from build123d import *

# Parameters (mm, degrees)
ESQUISSE2_R             = 5
BOSS_EXTRU_2_DEPTH      = 8
ESQUISSE3_W             = 10
ESQUISSE3_H             = 34.323
BOSS_EXTRU_3_DEPTH      = 6
ENL_V_MAT_EXTRU_1_REACH = 139.007
ESQUISSE4_R             = 4


with BuildPart() as part:
    # Esquisse2 → Boss.-Extru.2 (new body)
    with BuildSketch(Plane(origin=(0, 0, 0), x_dir=(-1, 0, 0), z_dir=(0, 0, 1))):
        Polygon((-45, 128.646), (-45, 0), (-5, 0), (0, 0), (0, 64.323), (0, 128.646), (-5.55, 128.646), align=None)
        with Locations(Location((-22.5, 10, 0), (0, 0, 180))):
            Circle(ESQUISSE2_R, mode=Mode.SUBTRACT)
        with Locations((-22.5, 118.646)):
            Circle(ESQUISSE2_R, mode=Mode.SUBTRACT)
    extrude(amount=BOSS_EXTRU_2_DEPTH)

    # Esquisse3 → Boss.-Extru.3 (add)
    with BuildSketch(Plane(origin=(0, 0, 0), x_dir=(-1, 0, 0), z_dir=(0, 0, -1))):
        with Locations((-22.5, -91.4845)):
            Rectangle(ESQUISSE3_W, ESQUISSE3_H)
        with Locations((-22.5, -37.1615)):
            Rectangle(ESQUISSE3_W, ESQUISSE3_H)
    extrude(amount=BOSS_EXTRU_3_DEPTH)

    # Esquisse4 → Enlèv. mat.-Extru.1 (cut, up to next)
    with BuildSketch(Plane.XY.offset(8), mode=Mode.PRIVATE) as enl_v_mat_extru_1_sk1:
        with Locations((10.1018, -28.6106)):
            Circle(ESQUISSE4_R)
    enl_v_mat_extru_1_tool1 = extrude(enl_v_mat_extru_1_sk1.sketch, amount=-ENL_V_MAT_EXTRU_1_REACH, mode=Mode.PRIVATE) & part.part
    # Esquisse4 → Enlèv. mat.-Extru.1 (cut, up to next)
    with BuildSketch(Plane.XY.offset(8), mode=Mode.PRIVATE) as enl_v_mat_extru_1_sk2:
        with Locations((10.1018, -100.0354)):
            Circle(ESQUISSE4_R)
    enl_v_mat_extru_1_tool2 = extrude(enl_v_mat_extru_1_sk2.sketch, amount=-ENL_V_MAT_EXTRU_1_REACH, mode=Mode.PRIVATE) & part.part
    # Esquisse4 → Enlèv. mat.-Extru.1 (cut, up to next)
    with BuildSketch(Plane.XY.offset(8), mode=Mode.PRIVATE) as enl_v_mat_extru_1_sk3:
        with Locations((18.84, -64.323)):
            Circle(ESQUISSE4_R)
    enl_v_mat_extru_1_tool3 = extrude(enl_v_mat_extru_1_sk3.sketch, amount=-ENL_V_MAT_EXTRU_1_REACH, mode=Mode.PRIVATE) & part.part
    add(enl_v_mat_extru_1_tool1.solids().sort_by_distance((10.1018, -28.6106, 8))[0], mode=Mode.SUBTRACT)
    add(enl_v_mat_extru_1_tool2.solids().sort_by_distance((10.1018, -100.0354, 8))[0], mode=Mode.SUBTRACT)
    add(enl_v_mat_extru_1_tool3.solids().sort_by_distance((18.84, -64.323, 8))[0], mode=Mode.SUBTRACT)


solid = part.part
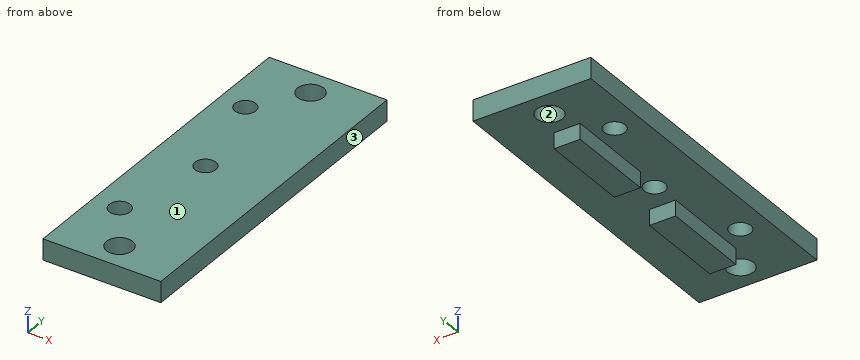
Work out the finished part from the listing and answer in its coordinate system (mm). Face numbers are marked on the shaded views. Round coordinates to 2 decimals unless told otherwise and drop trailing zeros. Order: outer loops, then holes, each group sorted by start corner. A loop starts at its lowest first (then second) coordinate and runs counter-clockwise, first axis right, second up. Notation, with made-up numbers: M 13,-16 L 52,-16 A27 ccw 52,9 Z; hole C 61,56.5 d5. An arc over 180 degrees is marked long. Put each result on its own line as item: value. Start each with the question number.
Q1. Section C-C, the plane y = -35 is taken. Write down the section's boundary in (x, z), and give its area (3 significant figures).
Q2. For a pull along X with two mould halves and no side action, classify the marked faces 1, 2 and 3 as pulls with the +X half, pulls with the -X half, needs draft (parallel to the pull), parting line crosses it, or undercut.
Q3. Section B-B, the plane x = 9 is taken. Write down the section's boundary in (y, z), and give its area (3 significant figures).
Q4. Section A-A, the plane y = -10 is taken. Write down the section's boundary in (x, z), and give its area (3 significant figures).
Q5. Flat-ended cylindrical pins translate along their axes: pin 1 (6.5 mm diameter, centred on y = -44, z = -4, fed in from +X); pin 2 (3 mm diameter, centred on y = -35.5, z = -2.5, fed in from -X); pin 3 (2 mm diameter, centred on x = 8, y = -47, fed in from -Z); pin 4 (10.5 mm diameter, centred on x = 10.1, y = -100.04, fed in from +Z). Find the tip coordinate at first contact, or state that the pin passes through.
Q6. Straight lines are drawn through the part: L1, parallel to Y at x = 18.84, z = 2.75; L2, parallel to Y at x = 13.5, z = 5; L3, parallel to Y at x = 22, z = 1.75. For each, find the intervals that lie inside material, in ascending order. Write a range as [from, to].
Q7. Section D-D, the plane x = 21.5 is taken. Write down the section's boundary in (y, z), and give its area (3 significant figures).
Findings below:
1. outline: M 0,0 L 17.5,0 L 17.5,-6 L 27.5,-6 L 27.5,0 L 45,0 L 45,8 L 0,8 Z
1. area: 420 mm^2
2. face 1: needs draft
2. face 2: undercut
2. face 3: pulls with the +X half
3. outline: M -128.65,0 L -103.88,0 L -103.88,8 L -128.65,8 Z; M -96.19,0 L -32.46,0 L -32.46,8 L -96.19,8 Z; M -24.77,0 L 0,0 L 0,8 L -24.77,8 Z
3. area: 906 mm^2
4. outline: M 0,0 L 17.5,0 L 17.5,8 L 0,8 Z; M 27.5,0 L 45,0 L 45,8 L 27.5,8 Z
4. area: 280 mm^2
5. pin 1: stops at x = 27.5
5. pin 2: stops at x = 17.5
5. pin 3: stops at z = 0
5. pin 4: stops at z = 8
6. L1: y = [-128.65, -122.05], [-115.24, -68.32], [-60.32, -13.41], [-6.59, 0]
6. L2: y = [-128.65, -102.15], [-97.93, -30.72], [-26.5, 0]
6. L3: y = [-128.65, -123.62], [-113.67, -66.78], [-61.87, -14.97], [-5.03, 0]
7. outline: M -128.65,0 L -123.54,0 L -123.54,8 L -128.65,8 Z; M -113.75,0 L -108.65,0 L -108.65,-6 L -74.32,-6 L -74.32,0 L -67.31,0 L -67.31,8 L -113.75,8 Z; M -61.34,0 L -54.32,0 L -54.32,-6 L -20,-6 L -20,0 L -14.9,0 L -14.9,8 L -61.34,8 Z; M -5.1,0 L 0,0 L 0,8 L -5.1,8 Z
7. area: 1,240 mm^2
